Input: part model. Units: mm. Frame: model coordinates. A direction names the side the tool comes from. Round coordinates to 2 decimals unless told otherwise and drop trailing zeros. Loops run counter-clockwise (first coordinate to the right, second up) from the corner with the lowest first, then second, coordinate; pieces in that order, holes last. Notation, with made-up numbers: (-0.75, 17.25) -> (31.25, 17.25) arc R22 ccw to (31.25, 31.25) -> close; hole circle Ø7 at (21.5, -22.75). An arc over 180 degrees is marked (long way). Answer as a JSON object with one key per item and string values.
```python
from build123d import *

# Parameters (mm, degrees)
SKETCH5_R           = 5
SKETCH5_R_2         = 1.5
BOSS_EXTRUDE2_DEPTH = 12
SKETCH6_W           = 1
SKETCH6_H           = 1
CUT_EXTRUDE4_DEPTH  = 12
SKETCH7_W           = 1
SKETCH7_H           = 1
CUT_EXTRUDE6_DEPTH  = 4
SKETCH8_W           = 3
SKETCH8_H           = 2
CUT_EXTRUDE7_DEPTH  = 15


with BuildPart() as part:
    # Sketch5 → Boss-Extrude2 (new body)
    with BuildSketch(Plane.XY):
        Circle(SKETCH5_R)
        Circle(SKETCH5_R_2, mode=Mode.SUBTRACT)
    extrude(amount=BOSS_EXTRUDE2_DEPTH)

    # Sketch6 → Cut-Extrude4 (cut)
    with BuildSketch(Plane.XY.offset(12)):
        with Locations((-1.5, 0)):
            Rectangle(SKETCH6_W, SKETCH6_H)
    extrude(amount=-CUT_EXTRUDE4_DEPTH, mode=Mode.SUBTRACT)

    # Sketch7 → Cut-Extrude6 (cut)
    with BuildSketch(Plane.XY.offset(12)):
        with Locations((-5, 0)):
            Rectangle(SKETCH7_W, SKETCH7_H)
    extrude(amount=-CUT_EXTRUDE6_DEPTH, mode=Mode.SUBTRACT)

    # Sketch8 → Cut-Extrude7 (cut)
    with BuildSketch(Plane(origin=(0, 0, 0), x_dir=(-1, 0, 0), z_dir=(0, 0, -1))):
        with Locations((5, 0)):
            Rectangle(SKETCH8_W, SKETCH8_H)
    extrude(amount=-CUT_EXTRUDE7_DEPTH, mode=Mode.SUBTRACT)


solid = part.part
```
1) Section C-C, the plane z = 10.5. Output: boundary loops of the cut face in (x, y), plus the area to 3 significant figures.
Output:
{"outline": "(-4.9, -1) arc R5 ccw (long way) to (-4.9, 1) -> (-3.5, 1) -> (-3.5, -1) -> close; hole (-2, -0.5) -> (-1.41, -0.5) arc R1.5 ccw (long way) to (-1.41, 0.5) -> (-2, 0.5) -> close", "area": "68.0 mm^2"}
2) Ray query, probe 1 along X at (y, z) = (0, 6); probe 2 along Y at (x, z) = (0, 4); probe 3 along Y at (x, z) = (-1.5, 1.75). Return the intervals inside material, ascending.
Output:
{"probe 1": "x = -3.5 to -2, 1.5 to 5", "probe 2": "y = -5 to -1.5, 1.5 to 5", "probe 3": "y = -4.77 to -0.5, 0.5 to 4.77"}
3) Draft query along Y for faces 1 (the face through (-2, 0, 6)), 2 (the face through (5, 0, 6)), 3 (the face through (0, -2, 0)). Return one class per face: +Y half, -Y half, draft (parallel to the pull), parting line (faces both ways), or undercut.
Output:
{"face 1": "undercut", "face 2": "parting line", "face 3": "draft"}
4) Reachability of faces 4 (the face through (-3.5, 0, 6)), 5 (the face through (0, -2, 12)) from +Z, -Z, +X, -X, +Y, -Y: full face, straight path, thin tool, end or side. Return the list, or none.
Output:
{"face 4": "+Z, -Z, -X", "face 5": "+Z, +X, -X, +Y, -Y"}
5) Section B-B, the plane y = 0. Output: boundary loops of the cut face in (x, z), plus the area to 3 significant figures.
Output:
{"outline": "(-3.5, 0) -> (-2, 0) -> (-2, 12) -> (-3.5, 12) -> close; (1.5, 0) -> (5, 0) -> (5, 12) -> (1.5, 12) -> close", "area": "60.0 mm^2"}
6) Section A-A, the plane x = 0. Output: boundary loops of the cut face in (y, z).
Output:
{"outline": "(-5, 0) -> (-1.5, 0) -> (-1.5, 12) -> (-5, 12) -> close; (1.5, 0) -> (5, 0) -> (5, 12) -> (1.5, 12) -> close"}
7) Section D-D, the plane y = 4. Output: boundary loops of the cut face in (x, z), plus the area to 3 significant figures.
Output:
{"outline": "(-3, 0) -> (3, 0) -> (3, 12) -> (-3, 12) -> close", "area": "72.0 mm^2"}
8) Contact query for flat-ended pins moving along their axis: P1, Ø5, axis at x = 0, y = 0, coming from the -Z side; P2, Ø3, axis at y = -3, z = 9, coming from the +X side; P3, Ø0.7, axis at x = -4.5, z = 6.5, coming from the -Y side; P4, Ø1, axis at y = 0, z = 5, coming from the -X side. Output: stop coordinate, or through.
Output:
{"P1": "stops at z = 0", "P2": "stops at x = 4.77", "P3": "stops at y = -2.79", "P4": "stops at x = -3.5"}
